For this review, use the dimensioned drawing (mm, ordinates from the lowest corner) and the shaded views. A direction names the side the tool comes from. Give positions to 0.01 mm unless a question says otherwise; leave off trailing zeros. Order: outer loops, then holes, each group sorted by start corner. A loop starts at its lowest first (then second) coordinate and runs counter-clockwise, first axis right, second up. Notation, with made-up numbers: (49.5, 42.5) - (64.5, 42.5) arc R12 ccw to (64.5, 61.5) - close; hole circle Ø11 at (55, 39.25). An arc over 180 degrees is marked (long way). Use a Markdown table: item, result. Add a question column.
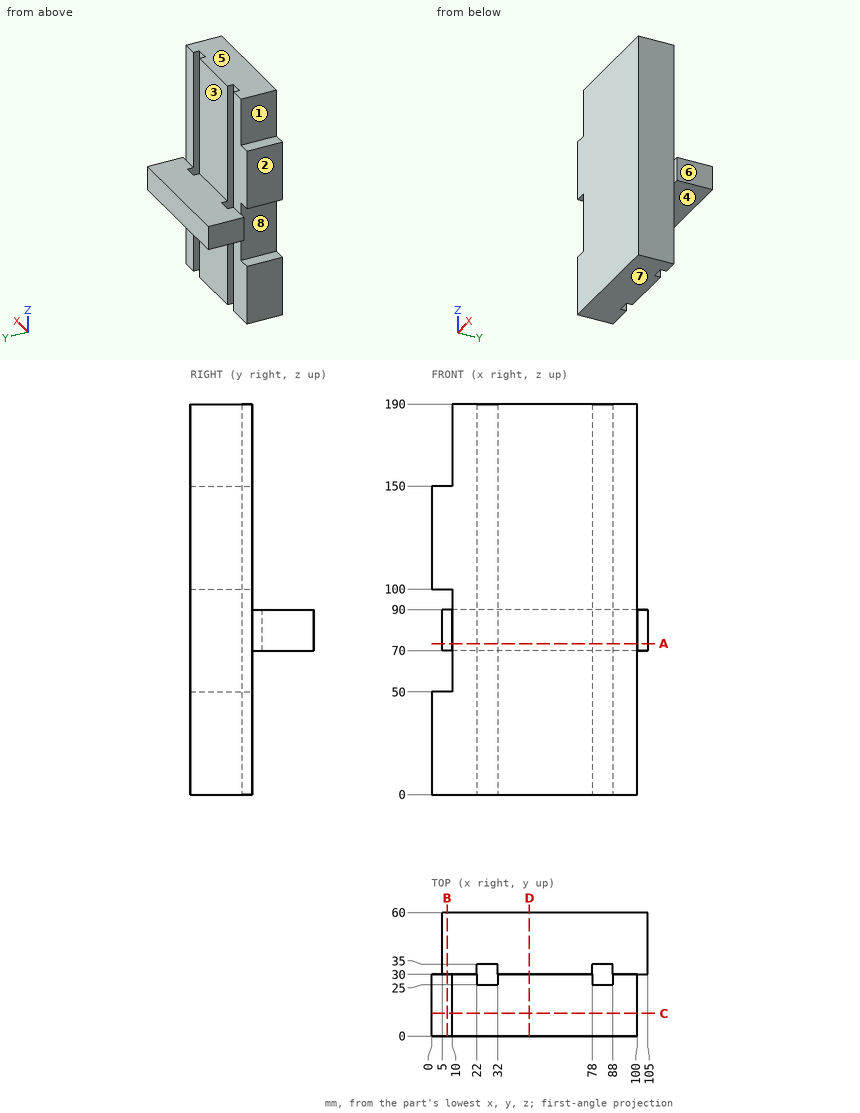
Q1. We need section C-C (y = 11). Write out the cut boundary in (x, z), plus the area to 3 significant figures.
Q2. Clearance check with flat-ended pins moving along their axes: P1, Ø17.5, axis at x = 16, z = 38, coming from the +Y side; P2, Ø3, axis at x = 72, y = 46.5, coming from the -Z side; P3, Ø8, axis at x = 3, y = 12.5, coming from the +Z side. State where each tip first meets the part, or that it passes through.
Q3. Wall thickness on probe 1 along X at (y, z) = (28, 118.5); probe 2 along Y at (x, z) = (23, 85); probe 3 along X at (y, z) = (23, 24): over which ranges is each line inside the solid? List them lowest first.
Q4. We need section B-B (x = 7.5). Write out the cut boundary in (y, z), plus the area to 3 significant figures.
Q5. Machinability: for the marked faces 1, 2, 3 and 4, which of the approach directions +Z, -Z, +X, -X, +Y, -Y give a long, thin tool a straight path to every point of the face, cutting with its end or side? Answer none if there is none.
Q6. We need section D-D (x = 47.5). Write out the cut boundary in (y, z).
Q7. We need section A-A (z = 73.5). Write out the cut boundary in (x, y), plus the area to 3 significant figures.
Q8. Draft analysis for pull direction Z (two halves, no side actions). For the marked faces 5, 6, 7 and 8, state which applies: pulls with the +Z half, pulls with the -Z half, needs draft (parallel to the pull), parting line crosses it, or undercut.
Here are the results:
| question | item | result |
|---|---|---|
| 1 | outline | (0, 0) - (100, 0) - (100, 190) - (10, 190) - (10, 150) - (0, 150) - (0, 100) - (10, 100) - (10, 50) - (0, 50) - close |
| 1 | area | 18,100 mm2 |
| 2 | P1 | y = 30 |
| 2 | P2 | z = 70 |
| 2 | P3 | z = 150 |
| 3 | probe 1 | 0 to 22, 32 to 78, 88 to 100 |
| 3 | probe 2 | 0 to 25, 35 to 60 |
| 3 | probe 3 | 0 to 100 |
| 4 | outline | (0, 0) - (30, 0) - (30, 50) - (0, 50) - close; (0, 100) - (30, 100) - (30, 150) - (0, 150) - close; (30, 70) - (60, 70) - (60, 90) - (30, 90) - close |
| 4 | area | 3,600 mm2 |
| 5 | face 1 | +Z, -X, +Y, -Y |
| 5 | face 2 | +Z, -Z, -X, +Y, -Y |
| 5 | face 3 | +Z, +X, -X, +Y |
| 5 | face 4 | -Z, +X, -X, +Y |
| 6 | outline | (0, 0) - (30, 0) - (30, 70) - (60, 70) - (60, 90) - (30, 90) - (30, 190) - (0, 190) - close |
| 7 | outline | (5, 30) - (10, 30) - (10, 0) - (100, 0) - (100, 30) - (105, 30) - (105, 60) - (5, 60) - close; hole (22, 25) - (32, 25) - (32, 35) - (22, 35) - close; hole (78, 25) - (88, 25) - (88, 35) - (78, 35) - close |
| 7 | area | 5,500 mm2 |
| 8 | face 5 | pulls with the +Z half |
| 8 | face 6 | needs draft |
| 8 | face 7 | pulls with the -Z half |
| 8 | face 8 | undercut |
